```python
from build123d import *

# Parameters (mm, degrees)
SKETCH1_W           = 70
SKETCH1_H           = 150
BOSS_EXTRUDE1_DEPTH = 5
SKETCH7_W           = 3.75
SKETCH7_H           = 30
BOSS_EXTRUDE2_DEPTH = 90
SKETCH10_W          = 60
SKETCH10_H          = 5
CUT_EXTRUDE2_DEPTH  = 75
SKETCH11_R          = 1.5
CUT_EXTRUDE3_DEPTH  = 75
CUT_EXTRUDE4_DEPTH  = 40
SKETCH13_R          = 1
SKETCH13_W          = 12
SKETCH13_H          = 22.5
CUT_EXTRUDE5_DEPTH  = 35


with BuildPart() as part:
    # Sketch1 → Boss-Extrude1 (new body)
    with BuildSketch(Plane(origin=(0, 0, 0), x_dir=(1, 0, 0), z_dir=(0, 1, 0))):
        Rectangle(SKETCH1_W, SKETCH1_H)
    extrude(amount=BOSS_EXTRUDE1_DEPTH)

    # Sketch7 → Boss-Extrude2 (add)
    with BuildSketch(Plane(origin=(0, 0, -75), x_dir=(-1, 0, 0), z_dir=(0, 0, -1))):
        with Locations((-33.125, 20)):
            Rectangle(SKETCH7_W, SKETCH7_H)
        with Locations((33.125, 20)):
            Rectangle(SKETCH7_W, SKETCH7_H)
    extrude(amount=-BOSS_EXTRUDE2_DEPTH)

    # Sketch10 → Cut-Extrude2 (cut)
    with BuildSketch(Plane(origin=(35, 0, 0), x_dir=(0, 0, -1), z_dir=(1, 0, 0))):
        with Locations((-45, 2.5)):
            Rectangle(SKETCH10_W, SKETCH10_H)
    extrude(amount=-CUT_EXTRUDE2_DEPTH, mode=Mode.SUBTRACT)

    # Sketch11 → Cut-Extrude3 (cut)
    with BuildSketch(Plane.ZY.offset(35)):
        with Locations((6, 20)):
            Circle(SKETCH11_R)
    extrude(amount=-CUT_EXTRUDE3_DEPTH, mode=Mode.SUBTRACT)

    # Sketch12 → Cut-Extrude4 (cut)
    with BuildSketch(Plane.XZ):
        Polygon((35, -75), (35, -21.162236792), (23.74549434, -21.162236792), (23.74549434, -49.878747724), (0, -49.878747724), (0, -75), (23.74549434, -75), align=None)
        Polygon((0, -75), (0, -49.878747724), (-23.74549434, -49.878747724), (-23.74549434, -21.162236792), (-35, -21.162236792), (-35, -75), (-23.74549434, -75), align=None)
    extrude(amount=-CUT_EXTRUDE4_DEPTH, mode=Mode.SUBTRACT)

    # Sketch13 → Cut-Extrude5 (cut)
    with BuildSketch(Plane.XZ):
        with Locations(Location((-10.75, 8.32, 0), (0, 0, 270))):
            Circle(SKETCH13_R)
        with Locations(Location((-10.75, -19, 0), (0, 0, 270))):
            Circle(SKETCH13_R)
        with Locations((-10.75, -5.34)):
            Rectangle(SKETCH13_W, SKETCH13_H)
    extrude(amount=-CUT_EXTRUDE5_DEPTH, mode=Mode.SUBTRACT)


solid = part.part
```
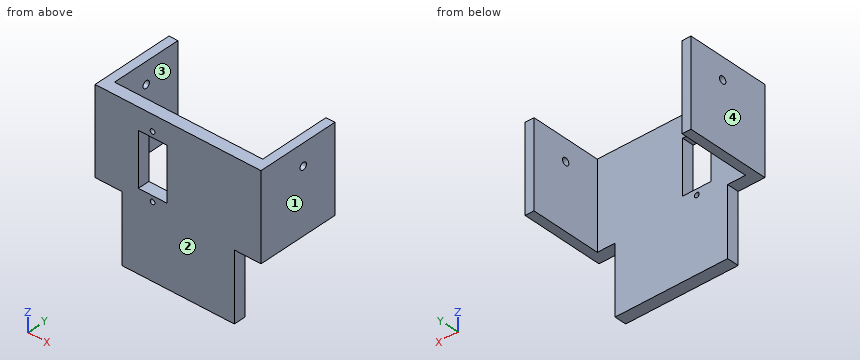
Geometry: final body of the model. Coordinates: model frame, mm. Face numbers are marked on the shaded views. Coordinates: 2 decimals unless noted, no trailing zeros. Order: outer loops, then holes, each group sorted by start corner. A loop starts at its lowest first (then second) coordinate and runs counter-clockwise, first axis right, second up. Notation, with made-up numbers: (14, 5) -> (31, 5) arc R19 cw to (31, 32) -> close; hole circle Ø1 at (45.5, -13.5). An arc over 180 degrees is marked (long way). Answer in a Markdown table with one row per item.
Item 1: Ray query, L1, parallel to X at y = 15, z = 7.5; L2, parallel to X at y = 2.05, z = -19; L3, parallel to Z at x = -10, y = 3. Return the intervals inside material, ascending.
Return value:
| item | result |
|---|---|
| L1 | x = -35 to -31.25, 31.25 to 35 |
| L2 | x = -35 to -11.75, -9.75 to 35 |
| L3 | z = -49.88 to -19.66, -18.34 to -16.59, 5.91 to 7.66, 8.98 to 15 |
Item 2: Section B-B on x = -10.75. Output: boundary loops of the cut face in (y, z).
Return value:
| item | result |
|---|---|
| outline | (0, -49.88) -> (5, -49.88) -> (5, -20) -> (0, -20) -> close; (0, -18) -> (5, -18) -> (5, -16.59) -> (0, -16.59) -> close; (0, 5.91) -> (5, 5.91) -> (5, 7.32) -> (0, 7.32) -> close; (0, 9.32) -> (5, 9.32) -> (5, 15) -> (0, 15) -> close |
Item 3: Contact query for flat-ended pins moving along their axis: P1, Ø5.5, axis at y = 3.5, z = -40, coming from the +X side; P2, Ø2.5, axis at y = 20, z = 6, coming from the +X side; P3, Ø4, axis at x = -12, z = -32, coming from the +Y side; P4, Ø5.5, axis at x = -30.5, y = 23, coming from the -Z side. Output: stop coordinate, or through.
Return value:
| item | result |
|---|---|
| P1 | stops at x = 23.75 |
| P2 | passes through |
| P3 | stops at y = 5 |
| P4 | stops at z = -21.16 |
Item 4: Section C-C on y = 20. Output: boundary loops of the cut face in (x, z), plus the area to 3 significant figures.
Return value:
| item | result |
|---|---|
| outline | (-35, -21.16) -> (-31.25, -21.16) -> (-31.25, 4.5) -> (-35, 4.5) -> close; (-35, 7.5) -> (-31.25, 7.5) -> (-31.25, 15) -> (-35, 15) -> close; (31.25, -21.16) -> (35, -21.16) -> (35, 4.5) -> (31.25, 4.5) -> close; (31.25, 7.5) -> (35, 7.5) -> (35, 15) -> (31.25, 15) -> close |
| area | 249 mm² |
Item 5: Section D-D on y = 8. Output: boundary loops of the cut face in (x, z).
Return value:
| item | result |
|---|---|
| outline | (-35, -21.16) -> (-31.25, -21.16) -> (-31.25, 15) -> (-35, 15) -> close; (31.25, -21.16) -> (35, -21.16) -> (35, 15) -> (31.25, 15) -> close |
Item 6: Draft query along X for the marked faces 1, 2, 3 and 4. Return one class per face: released by +X, released by -X, zero draft, split by the parting line, or undercut.
Return value:
| item | result |
|---|---|
| face 1 | released by +X |
| face 2 | zero draft |
| face 3 | undercut |
| face 4 | released by -X |
Item 7: Section A-A on z = -5. Output: boundary loops of the cut face in (x, y).
Return value:
| item | result |
|---|---|
| outline | (-35, 0) -> (-16.75, 0) -> (-16.75, 5) -> (-31.25, 5) -> (-31.25, 35) -> (-35, 35) -> close; (-4.75, 0) -> (35, 0) -> (35, 35) -> (31.25, 35) -> (31.25, 5) -> (-4.75, 5) -> close |
